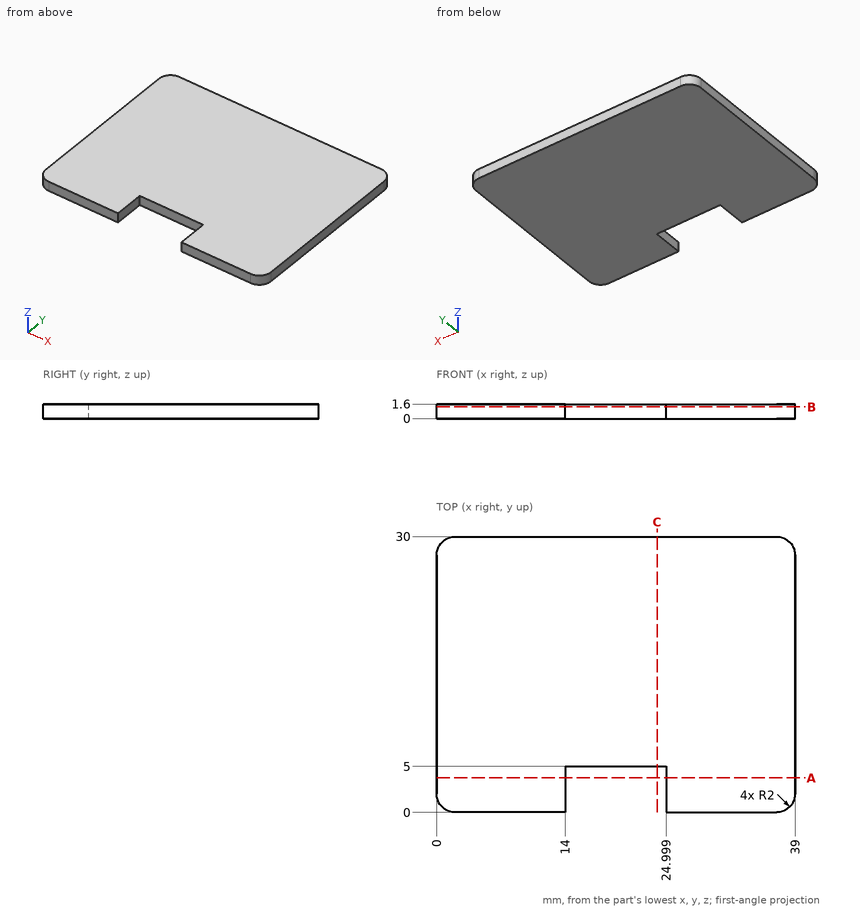
Study the drawing (mm; zero at the part's minimum x, y, z) and answer. Round coordinates to 2 decimals unless told otherwise and drop trailing zeros. Write each loop counter-clockwise with the first axis right and the second up, starting at its lowest first coordinate (ties: lowest second). Pieces come first, ordered by that corner, then holes.
1) A cutting plane is placed at B-B (z = 1.3). Give the vertices of the cut face in (x, y).
2) A cutting plane is placed at C-C (x = 24). Give the vertices of the cut face in (y, z).
3) Straight lines are drawn through the part: line 1 (X direction, y = 2.75, z = 1.15); line 2 (Y direction, x = 16, z = 1.3); line 3 (Y direction, x = 37.5, z = 1.3) (1 decimal). For each, find the intervals that lie inside material, in ascending order.
4) A cutting plane is placed at A-A (y = 3.75). Give the vertices of the cut face in (x, z).
5) Given pin 1 Ø0.8 at (x, z) = (22, 0.5) entering from -Y, flat-ended and moving along its own axis, determine where the tip first touches the part or whether it passes through.
Completed:
1. outline: (0, 2) arc R2 ccw to (2, 0) - (14, 0) - (14, 5) - (25, 5) - (25, 0) - (37, 0) arc R2 ccw to (39, 2) - (39, 28) arc R2 ccw to (37, 30) - (2, 30) arc R2 ccw to (0, 28) - close
2. outline: (5, 0) - (30, 0) - (30, 1.6) - (5, 1.6) - close
3. line 1: x = 0 to 14, 25 to 39
3. line 2: y = 5 to 30
3. line 3: y = 0.1 to 29.9
4. outline: (0, 0) - (14, 0) - (14, 1.6) - (0, 1.6) - close; (25, 0) - (39, 0) - (39, 1.6) - (25, 1.6) - close
5. pin 1: stops at y = 5
